```python
from build123d import *

# Parameters (mm, degrees)
SKETCH1_W           = 28.28
SKETCH1_H           = 327.5
BOSS_EXTRUDE1_DEPTH = 5
SKETCH2_R           = 2.1
CUT_EXTRUDE1_DEPTH  = 10
SKETCH3_R           = 2.1
CUT_EXTRUDE2_DEPTH  = 10


with BuildPart() as part:
    # Sketch1 → Boss-Extrude1 (new body)
    with BuildSketch(Plane.XY):
        Rectangle(SKETCH1_W, SKETCH1_H)
    extrude(amount=BOSS_EXTRUDE1_DEPTH)

    # Sketch2 → Cut-Extrude1 (cut)
    with BuildSketch(Plane.XY.offset(5)):
        with Locations((1.058524548, 96.25)):
            Circle(SKETCH2_R)
        Polygon((5, 163.75), (5, 153.75), (2.1, 153.75), (2.1, 148.75), (-2.1, 148.75), (-2.1, 153.75), (-5, 153.75), (-5, 163.75), align=None)
        Polygon((2.1, -148.75), (-2.1, -148.75), (-2.1, -153.75), (-5, -153.75), (-5, -163.75), (5, -163.75), (5, -153.75), (2.1, -153.75), align=None)
    extrude(amount=-CUT_EXTRUDE1_DEPTH, mode=Mode.SUBTRACT)

    # Sketch3 → Cut-Extrude2 (cut)
    with BuildSketch(Plane.XY.offset(5)):
        with Locations((-0.002135624, -101.25)):
            Circle(SKETCH3_R)
    extrude(amount=-CUT_EXTRUDE2_DEPTH, mode=Mode.SUBTRACT)


solid = part.part
```
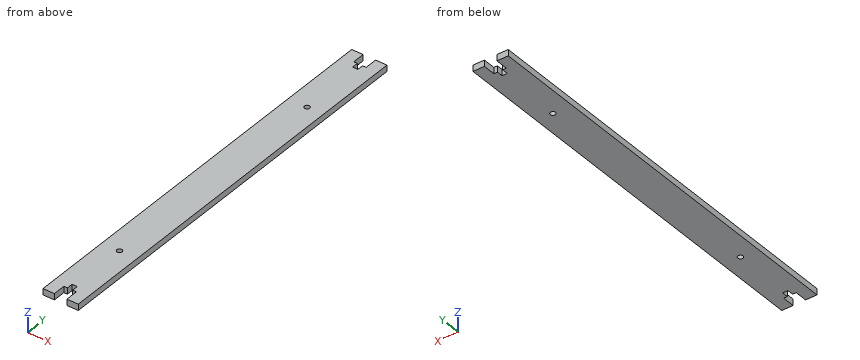
The listing builds one solid part. Answer for the finished solid, in the listing's coordinates (mm). Give positions to 0.01 mm unless a question says otherwise; leave off trailing zeros. Order: outer loops, then holes, each group sorted by start corner. A loop starts at its lowest first (then second) coordinate and runs counter-clockwise, first axis right, second up.
1) Consider line 1 along Y through (x, z) = (-2.75, 4.15); line 2 along X through (y, z) = (-150, 1.95); line 3 along Y through (x, z) = (2.25, 1.9). Determine where each line is inside the solid, lowest interval first.
Reported:
line 1: y = -153.75 to 153.75
line 2: x = -14.14 to -2.1, 2.1 to 14.14
line 3: y = -153.75 to 94.52, 97.98 to 153.75
2) Given P1, Ø1, axis at x = 7.5, y = -15, coming from the -Z side; P2, Ø0.9, axis at x = -3.5, z = 3.5, coming from the -Y side; P3, Ø2.5, axis at x = -3.5, z = 1.5, coming from the +Y side, each flat-ended and moving along its own axis, determine where each tip first touches the part or whether it passes through.
Reported:
P1: stops at z = 0
P2: stops at y = -153.75
P3: stops at y = 153.75
3) Find section A-A on z = 1.85. Write down the section's boundary in (x, y).
Reported:
outline: (-14.14, -163.75) - (-5, -163.75) - (-5, -153.75) - (-2.1, -153.75) - (-2.1, -148.75) - (2.1, -148.75) - (2.1, -153.75) - (5, -153.75) - (5, -163.75) - (14.14, -163.75) - (14.14, 163.75) - (5, 163.75) - (5, 153.75) - (2.1, 153.75) - (2.1, 148.75) - (-2.1, 148.75) - (-2.1, 153.75) - (-5, 153.75) - (-5, 163.75) - (-14.14, 163.75) - close; hole circle Ø4.2 at (0, -101.25); hole circle Ø4.2 at (1.06, 96.25)
